from build123d import *

# Parameters (mm, degrees)
BOSS_EXTRUDE1_DEPTH = 4.826


with BuildPart() as part:
    # Sketch1 → Boss-Extrude1 (new body)
    with BuildSketch(Plane.XY):
        with BuildLine():
            ThreePointArc((76.2, 25.4), (80.690128061, 23.540128061), (82.55, 19.05))
            Line((82.55, 19.05), (82.55, 12.7))
            Line((82.55, 12.7), (184.15, 12.7))
            Line((184.15, 12.7), (184.15, 19.05))
            ThreePointArc((184.15, 19.05), (186.009871939, 23.540128061), (190.5, 25.4))
            Line((190.5, 25.4), (260.35, 25.4))
            ThreePointArc((260.35, 25.4), (264.840128061, 23.540128061), (266.7, 19.05))
            Line((266.7, 19.05), (266.7, 6.35))
            ThreePointArc((266.7, 6.35), (264.840128061, 1.859871939), (260.35, 0))
            Line((260.35, 0), (6.35, 0))
            ThreePointArc((6.35, 0), (1.859871939, 1.859871939), (0, 6.35))
            Line((0, 6.35), (0, 19.05))
            ThreePointArc((0, 19.05), (1.859871939, 23.540128061), (6.35, 25.4))
            Line((6.35, 25.4), (76.2, 25.4))
        make_face()
    extrude(amount=BOSS_EXTRUDE1_DEPTH)


solid = part.part
Geometry check sheet. Reference: the model listing, model coordinates, mm. A direction names the side the tool comes from. Coordinates: 2 decimals unless noted, no trailing zeros. Order: outer loops, then holes, each group sorted by start corner. A loop starts at its lowest first (then second) coordinate and runs counter-clockwise, first axis right, second up. Notation, with made-up numbers: M 15,89 L 58,89 A20 ccw 58,112 Z; hole C 32,30 d7. An arc over 180 degrees is marked long. Use CSV: the item, a comma, the result in double quotes.
Item 1: Cross-section at D-D on x = 79. Record the cut outline in (y, z).
Returned:
outline,"M 0,0 L 24.75,0 L 24.75,4.83 L 0,4.83 Z"
Item 2: Cross-section at B-B on z = 2.05. Record the cut outline in (x, y).
Returned:
outline,"M 0,6.35 A6.35 ccw 6.35,0 L 260.35,0 A6.35 ccw 266.7,6.35 L 266.7,19.05 A6.35 ccw 260.35,25.4 L 190.5,25.4 A6.35 ccw 184.15,19.05 L 184.15,12.7 L 82.55,12.7 L 82.55,19.05 A6.35 ccw 76.2,25.4 L 6.35,25.4 A6.35 ccw 0,19.05 Z"
Item 3: Mould release check, pull along X, two halves, no side actions. Record for faces 1 (the cylindrical face through (264.89, 1.91, 2.38)), 2 (the flat face through (135, 10, 0)), 3 (the cylindrical face through (185.96, 23.49, 2.38)): pulls with the +X half, pulls with the -X half, needs draft (parallel to the pull), parting line crosses it, or undercut.
Returned:
face 1,"pulls with the +X half"
face 2,"needs draft"
face 3,"undercut"
Item 4: Gauge pin test, flat end, axial feed: pin 1 Ø1.4 at (x, z) = (140, 2) entering from +Y. Record the tip position at first contact, or that the pin passes through.
Returned:
pin 1,"stops at y = 12.7"
Item 5: Cross-section at A-A on y = 22. Record the cut outline in (x, z).
Returned:
outline,"M 0.73,0 L 81.82,0 L 81.82,4.83 L 0.73,4.83 Z; M 184.88,0 L 265.97,0 L 265.97,4.83 L 184.88,4.83 Z"
Item 6: Tool access check on faces 4 (the flat face through (266.7, 13, 2)), 5 (the flat face through (82.55, 16, 2)). Record the directions out of +Z, -Z, +X, -X, +Y, -Y that give a thin tool (end or side, any length) a straight path to the whole face; none if there is none.
Returned:
face 4,"+Z, -Z, +X, +Y, -Y"
face 5,"+Z, -Z, +Y"
Item 7: Thickness scan on line 1 along X through (y, z) = (17.25, 1.4); line 2 along Y through (x, z) = (100.5, 4.2); line 3 along X through (y, z) = (6.25, 0.95). Record the ranges inside material, lowest first.
Returned:
line 1,"x = 0 to 82.55, 184.15 to 266.7"
line 2,"y = 0 to 12.7"
line 3,"x = 0 to 266.7"
Item 8: Cross-section at C-C on x = 138.5. Record the cut outline in (y, z).
Returned:
outline,"M 0,0 L 12.7,0 L 12.7,4.83 L 0,4.83 Z"
